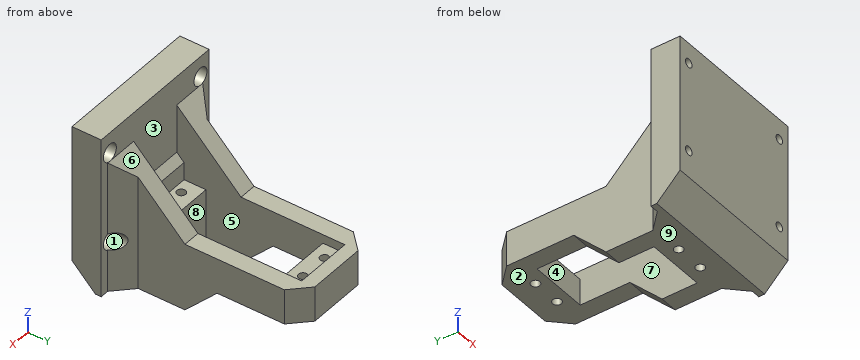
```python
from build123d import *

# Parameters (mm, degrees)
SKETCH1_W           = 50
SKETCH1_H           = 55
BOSS_EXTRUDE1_DEPTH = 10
SKETCH2_R           = 1.5
CUT_EXTRUDE1_DEPTH  = 4
CUT_EXTRUDE2_REACH  = 39.646
SKETCH3_R           = 3
SKETCH4_W           = 20
SKETCH4_H           = 20
BOSS_EXTRUDE2_DEPTH = 10
BOSS_EXTRUDE3_DEPTH = 6
SKETCH6_W           = 12
SKETCH6_H           = 12
BOSS_EXTRUDE4_DEPTH = 32
SKETCH7_W           = 20
SKETCH7_H           = 2.5
BOSS_EXTRUDE5_DEPTH = 6
SKETCH8_W           = 20
SKETCH8_H           = 7.5
CUT_EXTRUDE3_DEPTH  = 3
CHAMFER1_SIZE       = 2.5
CUT_EXTRUDE4_REACH  = 85.869
SKETCH9_R           = 1.5
CHAMFER3_SIZE       = 6
CHAMFER4_SIZE       = 8


# Some blends are built 0.0001 mm under size
with BuildPart() as part:
    # Sketch1 → Boss-Extrude1 (new body)
    with BuildSketch(Plane(origin=(0, 0, 0), x_dir=(1, 0, 0), z_dir=(0, 1, 0))):
        Rectangle(SKETCH1_W, SKETCH1_H)
    extrude(amount=BOSS_EXTRUDE1_DEPTH)

    # Sketch2 → Cut-Extrude1 (cut)
    with BuildSketch(Plane.XZ):
        with Locations(Location((-21, 20.5, 0), (0, 0, 270))):
            Circle(SKETCH2_R)
        with Locations(Location((21, 20.5, 0), (0, 0, 270))):
            Circle(SKETCH2_R)
        with Locations(Location((21, -10.2, 0), (0, 0, 270))):
            Circle(SKETCH2_R)
        with Locations(Location((-21, -10.2, 0), (0, 0, 270))):
            Circle(SKETCH2_R)
    extrude(amount=-CUT_EXTRUDE1_DEPTH, mode=Mode.SUBTRACT)

    # Sketch3 → Cut-Extrude2 (cut, up to next)
    with BuildSketch(Plane.XZ.offset(-4), mode=Mode.PRIVATE) as cut_extrude2_sk1:
        with Locations(Location((-21, 20.5, 0), (0, 0, 270))):
            Circle(SKETCH3_R)
    cut_extrude2_tool1 = extrude(cut_extrude2_sk1.sketch, amount=-CUT_EXTRUDE2_REACH, mode=Mode.PRIVATE) & part.part
    # Sketch3 → Cut-Extrude2 (cut, up to next)
    with BuildSketch(Plane.XZ.offset(-4), mode=Mode.PRIVATE) as cut_extrude2_sk2:
        with Locations(Location((21, 20.5, 0), (0, 0, 270))):
            Circle(SKETCH3_R)
    cut_extrude2_tool2 = extrude(cut_extrude2_sk2.sketch, amount=-CUT_EXTRUDE2_REACH, mode=Mode.PRIVATE) & part.part
    # Sketch3 → Cut-Extrude2 (cut, up to next)
    with BuildSketch(Plane.XZ.offset(-4), mode=Mode.PRIVATE) as cut_extrude2_sk3:
        with Locations(Location((21, -10.2, 0), (0, 0, 270))):
            Circle(SKETCH3_R)
    cut_extrude2_tool3 = extrude(cut_extrude2_sk3.sketch, amount=-CUT_EXTRUDE2_REACH, mode=Mode.PRIVATE) & part.part
    # Sketch3 → Cut-Extrude2 (cut, up to next)
    with BuildSketch(Plane.XZ.offset(-4), mode=Mode.PRIVATE) as cut_extrude2_sk4:
        with Locations(Location((-21, -10.2, 0), (0, 0, 270))):
            Circle(SKETCH3_R)
    cut_extrude2_tool4 = extrude(cut_extrude2_sk4.sketch, amount=-CUT_EXTRUDE2_REACH, mode=Mode.PRIVATE) & part.part
    add(cut_extrude2_tool1.solids().sort_by_distance((-21, 4, 20.5))[0], mode=Mode.SUBTRACT)
    add(cut_extrude2_tool2.solids().sort_by_distance((21, 4, 20.5))[0], mode=Mode.SUBTRACT)
    add(cut_extrude2_tool3.solids().sort_by_distance((21, 4, -10.2))[0], mode=Mode.SUBTRACT)
    add(cut_extrude2_tool4.solids().sort_by_distance((-21, 4, -10.2))[0], mode=Mode.SUBTRACT)

    # Sketch4 → Boss-Extrude2 (add)
    with BuildSketch(Plane(origin=(0, 10, 0), x_dir=(1, 0, 0), z_dir=(0, 1, 0))):
        with Locations((0, 17.5)):
            Rectangle(SKETCH4_W, SKETCH4_H)
    extrude(amount=BOSS_EXTRUDE2_DEPTH)

    # Sketch5 → Boss-Extrude3 (add)
    with BuildSketch(Plane(origin=(10, 0, 0), x_dir=(0, 0, -1), z_dir=(1, 0, 0))):
        Polygon((-17.5, 10), (4.5, 32), (4.5, 60), (16.5, 60), (16.5, 43), (27.5, 32), (27.5, 10), align=None)
    boss_extrude3 = extrude(amount=BOSS_EXTRUDE3_DEPTH)

    # Mirror1: Boss-Extrude3 across plane
    add(boss_extrude3.mirror(Plane(origin=(0, 0, 0), x_dir=(0, 0, 1), z_dir=(1, 0, 0))))

    # Sketch6 → Boss-Extrude4 (add)
    with BuildSketch(Plane(origin=(16, 0, 0), x_dir=(0, 0, -1), z_dir=(1, 0, 0))):
        with Locations((10.5, 66)):
            Rectangle(SKETCH6_W, SKETCH6_H)
    extrude(amount=-BOSS_EXTRUDE4_DEPTH)

    # Sketch7 → Boss-Extrude5 (add)
    with BuildSketch(Plane.XY.offset(-7.5)):
        with Locations((0, 11.25)):
            Rectangle(SKETCH7_W, SKETCH7_H)
    extrude(amount=BOSS_EXTRUDE5_DEPTH)

    # Sketch8 → Cut-Extrude3 (cut)
    with BuildSketch(Plane.XY.offset(-4.5)):
        with Locations((0, 63.75)):
            Rectangle(SKETCH8_W, SKETCH8_H)
    extrude(amount=-CUT_EXTRUDE3_DEPTH, mode=Mode.SUBTRACT)

    # Chamfer1
    chamfer1_edges = [part.edges().sort_by_distance(p)[0] for p in [
        (0, 10, -1.5),
    ]]
    chamfer(chamfer1_edges, length=CHAMFER1_SIZE - 0.0001)  # a hair under: the kernel refuses the full size

    # Sketch9 → Cut-Extrude4 (cut, up to next)
    with BuildSketch(Plane.XY.offset(-7.5), mode=Mode.PRIVATE) as cut_extrude4_sk1:
        with Locations((-5, 64.25)):
            Circle(SKETCH9_R)
    cut_extrude4_tool1 = extrude(cut_extrude4_sk1.sketch, amount=-CUT_EXTRUDE4_REACH, mode=Mode.PRIVATE) & part.part
    # Sketch9 → Cut-Extrude4 (cut, up to next)
    with BuildSketch(Plane.XY.offset(-7.5), mode=Mode.PRIVATE) as cut_extrude4_sk2:
        with Locations((5, 64.25)):
            Circle(SKETCH9_R)
    cut_extrude4_tool2 = extrude(cut_extrude4_sk2.sketch, amount=-CUT_EXTRUDE4_REACH, mode=Mode.PRIVATE) & part.part
    # Sketch9 → Cut-Extrude4 (cut, up to next)
    with BuildSketch(Plane.XY.offset(-7.5), mode=Mode.PRIVATE) as cut_extrude4_sk3:
        with Locations((5, 15.25)):
            Circle(SKETCH9_R)
    cut_extrude4_tool3 = extrude(cut_extrude4_sk3.sketch, amount=-CUT_EXTRUDE4_REACH, mode=Mode.PRIVATE) & part.part
    # Sketch9 → Cut-Extrude4 (cut, up to next)
    with BuildSketch(Plane.XY.offset(-7.5), mode=Mode.PRIVATE) as cut_extrude4_sk4:
        with Locations((-5, 15.25)):
            Circle(SKETCH9_R)
    cut_extrude4_tool4 = extrude(cut_extrude4_sk4.sketch, amount=-CUT_EXTRUDE4_REACH, mode=Mode.PRIVATE) & part.part
    add(cut_extrude4_tool1.solids().sort_by_distance((-5, 64.25, -7.5))[0], mode=Mode.SUBTRACT)
    add(cut_extrude4_tool2.solids().sort_by_distance((5, 64.25, -7.5))[0], mode=Mode.SUBTRACT)
    add(cut_extrude4_tool3.solids().sort_by_distance((5, 15.25, -7.5))[0], mode=Mode.SUBTRACT)
    add(cut_extrude4_tool4.solids().sort_by_distance((-5, 15.25, -7.5))[0], mode=Mode.SUBTRACT)

    # Chamfer3
    # the kernel refuses this chamfer: 6 mm, written as the material it adds along each edge
    with BuildSketch(Plane(origin=(16, 10, -27.5), x_dir=(0.9996219169112969, -0.02749587661058649, 0), z_dir=(0, 0, 1))) as chamfer3_piece_1_section:
        Polygon((CHAMFER3_SIZE * 0.999621916911, CHAMFER3_SIZE * 0.0274958766106), (-CHAMFER3_SIZE * 0.0274958766106, CHAMFER3_SIZE * 0.999621916911), (0, 0), align=None)
    chamfer3_piece_1 = extrude(amount=60.430097928, mode=Mode.PRIVATE)
    chamfer3_piece_1 = split(chamfer3_piece_1, bisect_by=Plane(origin=(17.926096491, 22.613963147, 4.886036853), z_dir=(0, -0.7071067811865474, -0.7071067811865478)), keep=Keep.TOP, mode=Mode.PRIVATE)
    chamfer3_piece_1 = chamfer3_piece_1 - Plane(origin=(21, 11.966350777, 20.5), x_dir=(0, 0, -1), z_dir=(0, -1, 0)) * Cylinder(3, 145, mode=Mode.PRIVATE)
    chamfer3_piece_1 = chamfer3_piece_1 - Plane(origin=(21, 11.966350777, -10.2), x_dir=(0, 0, -1), z_dir=(0, -1, 0)) * Cylinder(3, 145, mode=Mode.PRIVATE)
    add(chamfer3_piece_1)
    with BuildSketch(Plane(origin=(-16, 10, -27.5), x_dir=(-0.9996219169112969, -0.02749587661058649, 0), z_dir=(0, 0, 1))) as chamfer3_piece_2_section:
        Polygon((CHAMFER3_SIZE * 0.999621916911, -CHAMFER3_SIZE * 0.0274958766106), (-CHAMFER3_SIZE * 0.0274958766106, -CHAMFER3_SIZE * 0.999621916911), (0, 0), align=None)
    chamfer3_piece_2 = extrude(amount=60.430097928, mode=Mode.PRIVATE)
    chamfer3_piece_2 = split(chamfer3_piece_2, bisect_by=Plane(origin=(-17.926096431, 22.613963068, 4.886036932), z_dir=(0, -0.7071067811865474, -0.7071067811865478)), keep=Keep.TOP, mode=Mode.PRIVATE)
    chamfer3_piece_2 = chamfer3_piece_2 - Plane(origin=(-21, 11.966350831, 20.5), x_dir=(0, 0, -1), z_dir=(0, -1, 0)) * Cylinder(3, 145, mode=Mode.PRIVATE)
    chamfer3_piece_2 = chamfer3_piece_2 - Plane(origin=(-21, 11.966350831, -10.2), x_dir=(0, 0, -1), z_dir=(0, -1, 0)) * Cylinder(3, 145, mode=Mode.PRIVATE)
    add(chamfer3_piece_2)
    # the kernel refuses this chamfer: 6 mm, written as the material it takes off along each edge
    with BuildSketch(Plane(origin=(16, 72, -31.930097928), x_dir=(0.02749587661058648, -0.9996219169112968, 0), z_dir=(0, 0, 1)), Plane(origin=(-16, 72, -31.930097928), x_dir=(0.9996219169112968, 0.027495876610586775, 0), z_dir=(0, 0, 1))) as chamfer3_2_piece_1:
        Polygon((CHAMFER3_SIZE * 0.999621916911, -CHAMFER3_SIZE * 0.0274958766106), (-CHAMFER3_SIZE * 0.0274958766106, -CHAMFER3_SIZE * 0.999621916911), (0, 0), align=None)
    extrude(amount=42.860195856, mode=Mode.SUBTRACT)

    # Chamfer4
    chamfer4_edges = [part.edges().sort_by_distance(p)[0] for p in [
        (0, 0, -27.5),
    ]]
    chamfer(chamfer4_edges, length=CHAMFER4_SIZE)


solid = part.part
```
Check sheet for the modelled part. Datum: model origin and axes. Units: mm. Face numbers are marked on the shaded views. A direction names the side the tool comes from. Round coordinates to 2 decimals unless told otherwise and drop trailing zeros. Loops run counter-clockwise (first coordinate to the right, second up) from the corner with the lowest first, then second, coordinate; pieces in that order, holes last. Notation, with made-up numbers: (-5.5, 88) - (29.5, 88) arc R17 cw to (29.5, 109) - close; hole circle Ø11 at (-11, 55.5). An arc over 180 degrees is marked (long way). Write item = value, one per line. Start each with the question number.
Q1. Access from +Z, -Z, +X, -X, +Y, -Y to the whole of each face (thin tool, end or side, straight path). Record for the marked faces 1, 2, 3, 4 and 5.
Q2. Release check for a two-part mould opening along Y. For the marked faces 6, 7, 8 and 9 record: pulls with the +Y half, pulls with the -Y half, needs draft (parallel to the pull), parting line crosses it, or undercut.
Q3. Section check D-D (y = 64.25). Record the boundary of the cut face in (x, z), plus the area to 3 significant figures.
Q4. Thickness scan on L1, parallel to X at y = 1.6, z = -10.2; L2, parallel to X at y = 7, z = -10.2; L3, parallel to Y at x = 5, z = -12.75. Record the ranges inside material, lowest first.
Q5. Section check A-A (y = 46). Record the boundary of the cut face in (x, z), plus the area to 3 significant figures.
Q6. Section check B-B (x = -5). Count the separate pieces of the cut face and the enclosed holes in it, plus the area to 3 significant figures.
Q7. Section check C-C (y = 7). Record the boundary of the cut face in (x, z), plus the area to 3 significant figures.
Q8. Depth check by flat-ended pin: P1, Ø7, axis at x = 21, z = 20.5, coming from the +Y side; P2, Ø6, axis at x = -11.5, y = 53.5, coming from the +Z side; P3, Ø1.8, axis at x = -21, z = -10, coming from the +Y side; P4, Ø3.5, axis at x = -21, z = 20.5, coming from the +Y side. Enter the tip coordinate at first touch or a pass-through.
Derived:
q1.face_1 = +Y
q1.face_2 = -Z, +X, -X, +Y
q1.face_3 = +Z, +Y
q1.face_4 = +Z, -Z
q1.face_5 = +Z
q2.face_6 = pulls with the +Y half
q2.face_7 = undercut
q2.face_8 = undercut
q2.face_9 = needs draft
q3.outline = (-16, -16.5) - (-6.5, -16.5) - (-6.5, -7.5) - (-10, -7.5) - (-10, -4.5) - (-16, -4.5) - close; (-3.5, -16.5) - (3.5, -16.5) - (3.5, -7.5) - (-3.5, -7.5) - close; (6.5, -16.5) - (16, -16.5) - (16, -4.5) - (10, -4.5) - (10, -7.5) - (6.5, -7.5) - close
q3.area = 270 mm^2
q4.L1 = -25 to -22.5, -19.5 to 19.5, 22.5 to 25
q4.L2 = -25 to -24, -18 to 18, 24 to 25
q4.L3 = 0 to 13.75, 16.75 to 20, 60 to 62.75, 65.75 to 72
q5.outline = (-16, -16.5) - (-10, -16.5) - (-10, -4.5) - (-16, -4.5) - close; (10, -16.5) - (16, -16.5) - (16, -4.5) - (10, -4.5) - close
q5.area = 144 mm^2
q6.separate_pieces = 4
q6.enclosed_holes = 0
q6.area = 771 mm^2
q7.outline = (-25, -26.5) - (25, -26.5) - (25, 27.5) - (-25, 27.5) - close; hole circle Ø6 at (-21, -10.2); hole circle Ø6 at (-21, 20.5); hole circle Ø6 at (21, -10.2); hole circle Ø6 at (21, 20.5)
q7.area = 2,590 mm^2
q8.P1 = 10.5
q8.P2 = -4.5
q8.P3 = through
q8.P4 = 4
